from build123d import *

# Parameters (mm, degrees)
BOSS_EXTRUDE1_DEPTH = 3.81
BOSS_EXTRUDE2_DEPTH = 45.72
CUT_EXTRUDE1_REACH  = 100.694
SKETCH4_R           = 2.58
CUT_EXTRUDE2_REACH  = 150.732
CUT_EXTRUDE3_REACH  = 147.358
SKETCH8_R           = 1.085
SKETCH10_W          = 6.281419417
SKETCH10_H          = 8.338567611
SKETCH10_W_2        = 6.611751911
SKETCH10_H_2        = 8.662901092
CUT_EXTRUDE4_DEPTH  = 1.524
BOSS_EXTRUDE3_DEPTH = 10.16
SKETCH12_R          = 2.447521694
SKETCH12_R_2        = 2.570723965
SKETCH12_R_3        = 2.649131916
SKETCH12_R_4        = 2.514751493
CUT_EXTRUDE5_DEPTH  = 5.08


with BuildPart() as part:
    # Sketch1 → Boss-Extrude1 (new body)
    with BuildSketch(Plane.XY):
        with BuildLine():
            Line((66.150214266, -46.99), (-66.150214266, -46.99))
            ThreePointArc((-66.150214266, -46.99), (-71.538367938, -44.758153673), (-73.770214266, -39.37))
            Line((-73.770214266, -39.37), (-73.770214266, 39.37))
            ThreePointArc((-73.770214266, 39.37), (-71.538367938, 44.758153673), (-66.150214266, 46.99))
            Line((-66.150214266, 46.99), (66.150214266, 46.99))
            ThreePointArc((66.150214266, 46.99), (71.538367938, 44.758153673), (73.770214266, 39.37))
            Line((73.770214266, 39.37), (73.770214266, -39.37))
            ThreePointArc((73.770214266, -39.37), (71.538367938, -44.758153673), (66.150214266, -46.99))
        make_face()
        with BuildLine():
            Line((45.974935849, -43.18), (-45.974935849, -43.18))
            ThreePointArc((-45.974935849, -43.18), (-51.363089522, -40.948153673), (-53.594935849, -35.56))
            Line((-53.594935849, -35.56), (-53.594935849, 35.56))
            ThreePointArc((-53.594935849, 35.56), (-51.363089522, 40.948153673), (-45.974935849, 43.18))
            Line((-45.974935849, 43.18), (45.974935849, 43.18))
            ThreePointArc((45.974935849, 43.18), (51.363089522, 40.948153673), (53.594935849, 35.56))
            Line((53.594935849, 35.56), (53.594935849, -35.56))
            ThreePointArc((53.594935849, -35.56), (51.363089522, -40.948153673), (45.974935849, -43.18))
        make_face(mode=Mode.SUBTRACT)
    extrude(amount=BOSS_EXTRUDE1_DEPTH)

    # Sketch2 → Boss-Extrude2 (add)
    with BuildSketch(Plane.XY.offset(3.81)):
        with BuildLine():
            Line((50.745873235, -46.99), (-50.745873235, -46.99))
            ThreePointArc((-50.745873235, -46.99), (-56.134026908, -44.758153673), (-58.365873235, -39.37))
            Line((-58.365873235, -39.37), (-58.365873235, 39.37))
            ThreePointArc((-58.365873235, 39.37), (-56.134026908, 44.758153673), (-50.745873235, 46.99))
            Line((-50.745873235, 46.99), (50.745873235, 46.99))
            ThreePointArc((50.745873235, 46.99), (56.134026908, 44.758153673), (58.365873235, 39.37))
            Line((58.365873235, 39.37), (58.365873235, -39.37))
            ThreePointArc((58.365873235, -39.37), (56.134026908, -44.758153673), (50.745873235, -46.99))
        make_face()
        with BuildLine():
            Line((46.935873235, -43.18), (-46.935873235, -43.18))
            ThreePointArc((-46.935873235, -43.18), (-52.324026908, -40.948153673), (-54.555873235, -35.56))
            Line((-54.555873235, -35.56), (-54.555873235, 35.56))
            ThreePointArc((-54.555873235, 35.56), (-52.324026908, 40.948153673), (-46.935873235, 43.18))
            Line((-46.935873235, 43.18), (46.935873235, 43.18))
            ThreePointArc((46.935873235, 43.18), (52.324026908, 40.948153673), (54.555873235, 35.56))
            Line((54.555873235, 35.56), (54.555873235, -35.56))
            ThreePointArc((54.555873235, -35.56), (52.324026908, -40.948153673), (46.935873235, -43.18))
        make_face(mode=Mode.SUBTRACT)
    extrude(amount=BOSS_EXTRUDE2_DEPTH)

    # Sketch4 → Cut-Extrude1 (cut, up to next)
    with BuildSketch(Plane.XY.offset(3.81), mode=Mode.PRIVATE) as cut_extrude1_sk1:
        with Locations((61.206014266, 22.22917718)):
            Circle(SKETCH4_R)
    cut_extrude1_tool1 = extrude(cut_extrude1_sk1.sketch, amount=-CUT_EXTRUDE1_REACH, mode=Mode.PRIVATE) & part.part
    # Sketch4 → Cut-Extrude1 (cut, up to next)
    with BuildSketch(Plane.XY.offset(3.81), mode=Mode.PRIVATE) as cut_extrude1_sk2:
        with Locations((61.206005964, -22.22082282)):
            Circle(SKETCH4_R)
    cut_extrude1_tool2 = extrude(cut_extrude1_sk2.sketch, amount=-CUT_EXTRUDE1_REACH, mode=Mode.PRIVATE) & part.part
    # Sketch4 → Cut-Extrude1 (cut, up to next)
    with BuildSketch(Plane.XY.offset(3.81), mode=Mode.PRIVATE) as cut_extrude1_sk3:
        with Locations((-60.973994036, -22.2208)):
            Circle(SKETCH4_R)
    cut_extrude1_tool3 = extrude(cut_extrude1_sk3.sketch, amount=-CUT_EXTRUDE1_REACH, mode=Mode.PRIVATE) & part.part
    # Sketch4 → Cut-Extrude1 (cut, up to next)
    with BuildSketch(Plane.XY.offset(3.81), mode=Mode.PRIVATE) as cut_extrude1_sk4:
        with Locations((-60.973985734, 22.2292)):
            Circle(SKETCH4_R)
    cut_extrude1_tool4 = extrude(cut_extrude1_sk4.sketch, amount=-CUT_EXTRUDE1_REACH, mode=Mode.PRIVATE) & part.part
    add(cut_extrude1_tool1.solids().sort_by_distance((61.206014, 22.229177, 3.81))[0], mode=Mode.SUBTRACT)
    add(cut_extrude1_tool2.solids().sort_by_distance((61.206006, -22.220823, 3.81))[0], mode=Mode.SUBTRACT)
    add(cut_extrude1_tool3.solids().sort_by_distance((-60.973994, -22.2208, 3.81))[0], mode=Mode.SUBTRACT)
    add(cut_extrude1_tool4.solids().sort_by_distance((-60.973986, 22.2292, 3.81))[0], mode=Mode.SUBTRACT)

    # Sketch7 → Cut-Extrude2 (cut, up to next)
    with BuildSketch(Plane.ZY.offset(58.365873235), mode=Mode.PRIVATE) as cut_extrude2_sk1:
        with BuildLine():
            Line((11.791283781, 13.03362733), (11.791283781, -18.68237267))
            ThreePointArc((11.791283781, -18.68237267), (13.502365966, -22.813290486), (17.633283781, -24.52437267))
            Line((17.633283781, -24.52437267), (29.481979429, -24.52437267))
            ThreePointArc((29.481979429, -24.52437267), (33.612897244, -22.813290486), (35.323979429, -18.68237267))
            Line((35.323979429, -18.68237267), (35.323979429, 13.03362733))
            ThreePointArc((35.323979429, 13.03362733), (33.612897244, 17.164545145), (29.481979429, 18.87562733))
            Line((29.481979429, 18.87562733), (17.633283781, 18.87562733))
            ThreePointArc((17.633283781, 18.87562733), (13.502365966, 17.164545145), (11.791283781, 13.03362733))
        make_face()
    cut_extrude2_tool1 = extrude(cut_extrude2_sk1.sketch, amount=-CUT_EXTRUDE2_REACH, mode=Mode.PRIVATE) & part.part
    add(cut_extrude2_tool1.solids().sort_by_distance((-58.365873, -2.824373, 23.557632))[0], mode=Mode.SUBTRACT)

    # Sketch8 → Cut-Extrude3 (cut, up to next)
    with BuildSketch(Plane(origin=(-54.555873235, 0, 0), x_dir=(0, 0, -1), z_dir=(1, 0, 0)), mode=Mode.PRIVATE) as cut_extrude3_sk1:
        with Locations(Location((-34.323979429, -26.52437267, 0), (0, 0, 90))):
            Circle(SKETCH8_R)
    cut_extrude3_tool1 = extrude(cut_extrude3_sk1.sketch, amount=-CUT_EXTRUDE3_REACH, mode=Mode.PRIVATE) & part.part
    # Sketch8 → Cut-Extrude3 (cut, up to next)
    with BuildSketch(Plane(origin=(-54.555873235, 0, 0), x_dir=(0, 0, -1), z_dir=(1, 0, 0)), mode=Mode.PRIVATE) as cut_extrude3_sk2:
        with Locations(Location((-16.223979429, -28.02437267, 0), (0, 0, 90))):
            Circle(SKETCH8_R)
    cut_extrude3_tool2 = extrude(cut_extrude3_sk2.sketch, amount=-CUT_EXTRUDE3_REACH, mode=Mode.PRIVATE) & part.part
    # Sketch8 → Cut-Extrude3 (cut, up to next)
    with BuildSketch(Plane(origin=(-54.555873235, 0, 0), x_dir=(0, 0, -1), z_dir=(1, 0, 0)), mode=Mode.PRIVATE) as cut_extrude3_sk3:
        with Locations(Location((-16.223979429, 22.37562733, 0), (0, 0, 90))):
            Circle(SKETCH8_R)
    cut_extrude3_tool3 = extrude(cut_extrude3_sk3.sketch, amount=-CUT_EXTRUDE3_REACH, mode=Mode.PRIVATE) & part.part
    # Sketch8 → Cut-Extrude3 (cut, up to next)
    with BuildSketch(Plane(origin=(-54.555873235, 0, 0), x_dir=(0, 0, -1), z_dir=(1, 0, 0)), mode=Mode.PRIVATE) as cut_extrude3_sk4:
        with Locations(Location((-34.323979429, 20.87562733, 0), (0, 0, 90))):
            Circle(SKETCH8_R)
    cut_extrude3_tool4 = extrude(cut_extrude3_sk4.sketch, amount=-CUT_EXTRUDE3_REACH, mode=Mode.PRIVATE) & part.part
    add(cut_extrude3_tool1.solids().sort_by_distance((-54.555873, -26.524373, 34.323979))[0], mode=Mode.SUBTRACT)
    add(cut_extrude3_tool2.solids().sort_by_distance((-54.555873, -28.024373, 16.223979))[0], mode=Mode.SUBTRACT)
    add(cut_extrude3_tool3.solids().sort_by_distance((-54.555873, 22.375627, 16.223979))[0], mode=Mode.SUBTRACT)
    add(cut_extrude3_tool4.solids().sort_by_distance((-54.555873, 20.875627, 34.323979))[0], mode=Mode.SUBTRACT)

    # Sketch10 → Cut-Extrude4 (cut)
    with BuildSketch(Plane.ZY.offset(58.365873235)):
        with Locations((6.950709709, 22.241628059)):
            Rectangle(SKETCH10_W, SKETCH10_H)
        with Locations((7.115875956, -22.482023984)):
            Rectangle(SKETCH10_W_2, SKETCH10_H_2)
    cut_extrude4 = extrude(amount=-CUT_EXTRUDE4_DEPTH, mode=Mode.SUBTRACT)

    # Mirror1: Cut-Extrude4 across plane
    add(cut_extrude4.mirror(Plane.ZY), mode=Mode.SUBTRACT)

    # Sketch11 → Boss-Extrude3 (add)
    with BuildSketch(Plane.XY.offset(49.53)):
        with BuildLine():
            Line((55.90804375, -54.61), (-55.90804375, -54.61))
            ThreePointArc((-55.90804375, -54.61), (-63.092248647, -51.634204897), (-66.06804375, -44.45))
            Line((-66.06804375, -44.45), (-66.06804375, 44.45))
            ThreePointArc((-66.06804375, 44.45), (-63.092248647, 51.634204897), (-55.90804375, 54.61))
            Line((-55.90804375, 54.61), (55.90804375, 54.61))
            ThreePointArc((55.90804375, 54.61), (63.092248647, 51.634204897), (66.06804375, 44.45))
            Line((66.06804375, 44.45), (66.06804375, -44.45))
            ThreePointArc((66.06804375, -44.45), (63.092248647, -51.634204897), (55.90804375, -54.61))
        make_face()
        with BuildLine():
            Line((50.82804375, -46.99), (-50.82804375, -46.99))
            ThreePointArc((-50.82804375, -46.99), (-56.216197423, -44.758153673), (-58.44804375, -39.37))
            Line((-58.44804375, -39.37), (-58.44804375, 39.37))
            ThreePointArc((-58.44804375, 39.37), (-56.216197423, 44.758153673), (-50.82804375, 46.99))
            Line((-50.82804375, 46.99), (50.82804375, 46.99))
            ThreePointArc((50.82804375, 46.99), (56.216197423, 44.758153673), (58.44804375, 39.37))
            Line((58.44804375, 39.37), (58.44804375, -39.37))
            ThreePointArc((58.44804375, -39.37), (56.216197423, -44.758153673), (50.82804375, -46.99))
        make_face(mode=Mode.SUBTRACT)
    extrude(amount=-BOSS_EXTRUDE3_DEPTH)

    # Sketch12 → Cut-Extrude5 (cut)
    with BuildSketch(Plane.XY.offset(49.53)):
        with Locations((-55.90804375, 46.99)):
            Circle(SKETCH12_R)
        with Locations((56.134026908, -44.758153673)):
            Circle(SKETCH12_R_2)
        with Locations((-56.216197423, -44.758153673)):
            Circle(SKETCH12_R_3)
        with Locations((56.134026908, 46.99)):
            Circle(SKETCH12_R_4)
    extrude(amount=-CUT_EXTRUDE5_DEPTH, mode=Mode.SUBTRACT)


solid = part.part
Build history of the part. All positions in model axes, mm. A direction names the side the tool comes from. Coordinates: 2 decimals unless noted, no trailing zeros. Order: outer loops, then holes, each group sorted by start corner. A loop starts at its lowest first (then second) coordinate and runs counter-clockwise, first axis right, second up. Notation, with made-up numbers: (62, -19.5) -> (91, -19.5) arc R30 cw to (91, 19.5) -> close; hole circle Ø2 at (86, -40). An arc over 180 degrees is marked (long way). One line per item, written item: value.
(1) Drop flat-ended pins along their axis: pin 1 Ø8 at (x, z) = (-3.5, 25) entering from +Y; pin 2 Ø0.5 at (x, z) = (-58, 5.5) entering from +Y; pin 3 Ø1.7 at (x, z) = (-57.5, 8) entering from -Y. Give the stop position or say it passes through.
Checked values:
pin 1: y = 46.99
pin 2: y = 42.37
pin 3: y = -44.19
(2) Tool access for faces 1 (the cylindrical face through (-56.488, 17.119, 33.658)), 2 (the cylindrical face through (-63.02, 20.66, 1.93)), 3 (the flat face through (-56, 47, 44.45)): list every direction of +Z, -Z, +X, -X, +Y, -Y with a clear straight run to the whole face (end or side of a thin tool).
Checked values:
face 1: -X
face 2: -Z
face 3: +Z
(3) Slice it at B-B, the plane z = 20.5. List the corners of the cut face in (x, y), plus the area to 3 significant figures.
Checked values:
outline: (-58.37, -39.37) arc R7.62 ccw to (-50.75, -46.99) -> (50.75, -46.99) arc R7.62 ccw to (58.37, -39.37) -> (58.37, 39.37) arc R7.62 ccw to (50.75, 46.99) -> (-50.75, 46.99) arc R7.62 ccw to (-58.37, 39.37) -> (-58.37, 18.88) -> (-54.56, 18.88) -> (-54.56, 35.56) arc R7.62 cw to (-46.94, 43.18) -> (46.94, 43.18) arc R7.62 cw to (54.56, 35.56) -> (54.56, -35.56) arc R7.62 cw to (46.94, -43.18) -> (-46.94, -43.18) arc R7.62 cw to (-54.56, -35.56) -> (-54.56, -24.52) -> (-58.37, -24.52) -> close
area: 1,380 mm2
(4) Probe line 1 (Y direction, x = -10, z = 35); line 2 (X direction, y = -30.5, z = 27); line 3 (X direction, y = 46, z = 46). List the from-to ranges inside material, lowest first. Write a range as [from, to].
Checked values:
line 1: [-46.99, -43.18], [43.18, 46.99]
line 2: [-58.37, -54.56], [54.56, 58.37]
line 3: [-65.95, -58.15], [-53.67, 53.82], [58.45, 65.95]
(5) Mould opens along X. For faces 4 (the cylindrical face through (57.64, 49.004, 47.026)), 5 (the cylindrical face through (63.013, 51.713, 44.521)), 6 (the cylindrical face through (52.26, 41.01, 26.35)), 7 (the flat face through (1, -48, 49.53)) say: pulls with the +X half, pulls with the -X half, needs draft (parallel to the pull), parting line crosses it, or undercut.
Checked values:
face 4: undercut
face 5: pulls with the +X half
face 6: undercut
face 7: needs draft
(6) Slice it at A-A, the plane y = -16.5. List the corners of the cut face in (x, z).
Checked values:
outline: (-73.77, 0) -> (-53.59, 0) -> (-53.59, 3.81) -> (-54.56, 3.81) -> (-54.56, 11.79) -> (-58.37, 11.79) -> (-58.37, 3.81) -> (-73.77, 3.81) -> close; (-66.07, 39.37) -> (-58.45, 39.37) -> (-58.45, 49.53) -> (-66.07, 49.53) -> close; (-58.37, 35.32) -> (-54.56, 35.32) -> (-54.56, 49.53) -> (-58.37, 49.53) -> close; (53.59, 0) -> (73.77, 0) -> (73.77, 3.81) -> (58.37, 3.81) -> (58.37, 49.53) -> (54.56, 49.53) -> (54.56, 3.81) -> (53.59, 3.81) -> close; (58.45, 39.37) -> (66.07, 39.37) -> (66.07, 49.53) -> (58.45, 49.53) -> close
